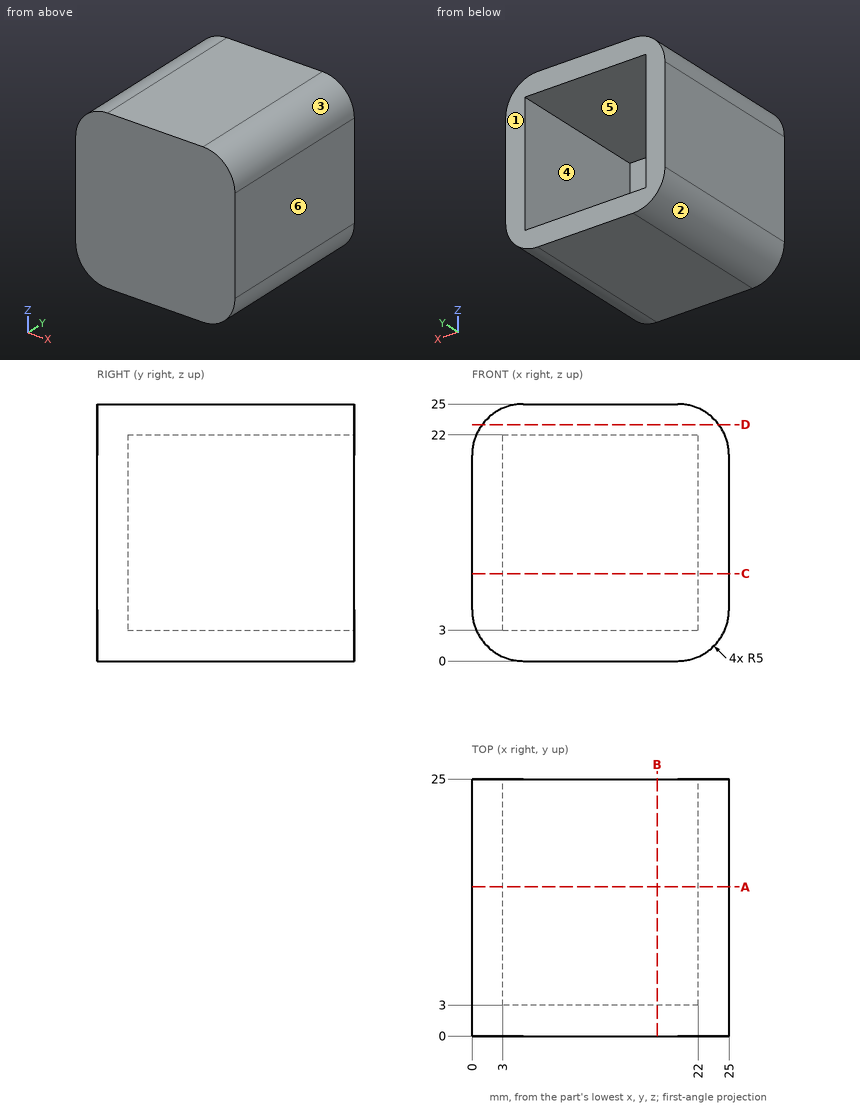
Geometry check sheet. Reference: drawing and pictorial views, mm from the part's lowest x, y, z. A direction names the side the tool comes from. Round coordinates to 2 decimals unless told otherwise and drop trailing zeros. Loops run counter-clockwise (first coordinate to the right, second up) from the corner with the lowest first, then second, coordinate; pieces in that order, holes last. Notation, with made-up numbers: (-2, 70.5) - (38, 70.5) arc R26 ccw to (38, 92.5) - close; hole circle Ø4 at (88.5, -7.5). An arc over 180 degrees is marked (long way). Answer as CSV lines item,"result".
(1) Depth check by flat-ended pin: pin 1 Ø15 at (x, z) = (14, 9.5) entering from +Y. Enter the tip coordinate at first touch or a pass-through.
Output values:
pin 1,"stops at y = 25"
(2) Cross-section at C-C, the plane z = 8.5. Enter the section's corners in (x, y), and give its area (3 significant figures).
Output values:
outline,"(0, 0) - (25, 0) - (25, 25) - (22, 25) - (22, 3) - (3, 3) - (3, 25) - (0, 25) - close"
area,"207 mm²"
(3) Release check for a two-part mould opening along X. For the marked faces 1, 2, 3 and 4 record: released by +X, released by -X, zero draft, split by the parting line, or undercut.
Output values:
face 1,"zero draft"
face 2,"released by -X"
face 3,"released by +X"
face 4,"undercut"
(4) Cross-section at A-A, the plane y = 14.5. Enter the section's corners in (x, z).
Output values:
outline,"(0, 5) arc R5 ccw to (5, 0) - (20, 0) arc R5 ccw to (25, 5) - (25, 20) arc R5 ccw to (20, 25) - (5, 25) arc R5 ccw to (0, 20) - close; hole (3, 3) - (22, 3) - (22, 22) - (3, 22) - close"
(5) Set-up check for the marked faces 5 and 6: record each of +Z, -Z, +X, -X, +Y, -Y from which the full face is reachable in a straight line by a thin tool's end or side.
Output values:
face 5,"+Y"
face 6,"+Z, -Z, +X, +Y, -Y"
(6) Cross-section at D-D, the plane z = 23. Enter the section's corners in (x, y).
Output values:
outline,"(1, 0) - (24, 0) - (24, 25) - (1, 25) - close"
(7) Cross-section at B-B, the plane x = 18. Enter the section's corners in (y, z).
Output values:
outline,"(0, 0) - (25, 0) - (25, 3) - (3, 3) - (3, 22) - (25, 22) - (25, 25) - (0, 25) - close"
(8) Material ranges on line 1 along Z through (x, y) = (17.5, 11.75); line 2 along Y through (x, z) = (5.75, 14.5), recorded low to high.
Output values:
line 1,"z = 0 to 3, 22 to 25"
line 2,"y = 0 to 3"
